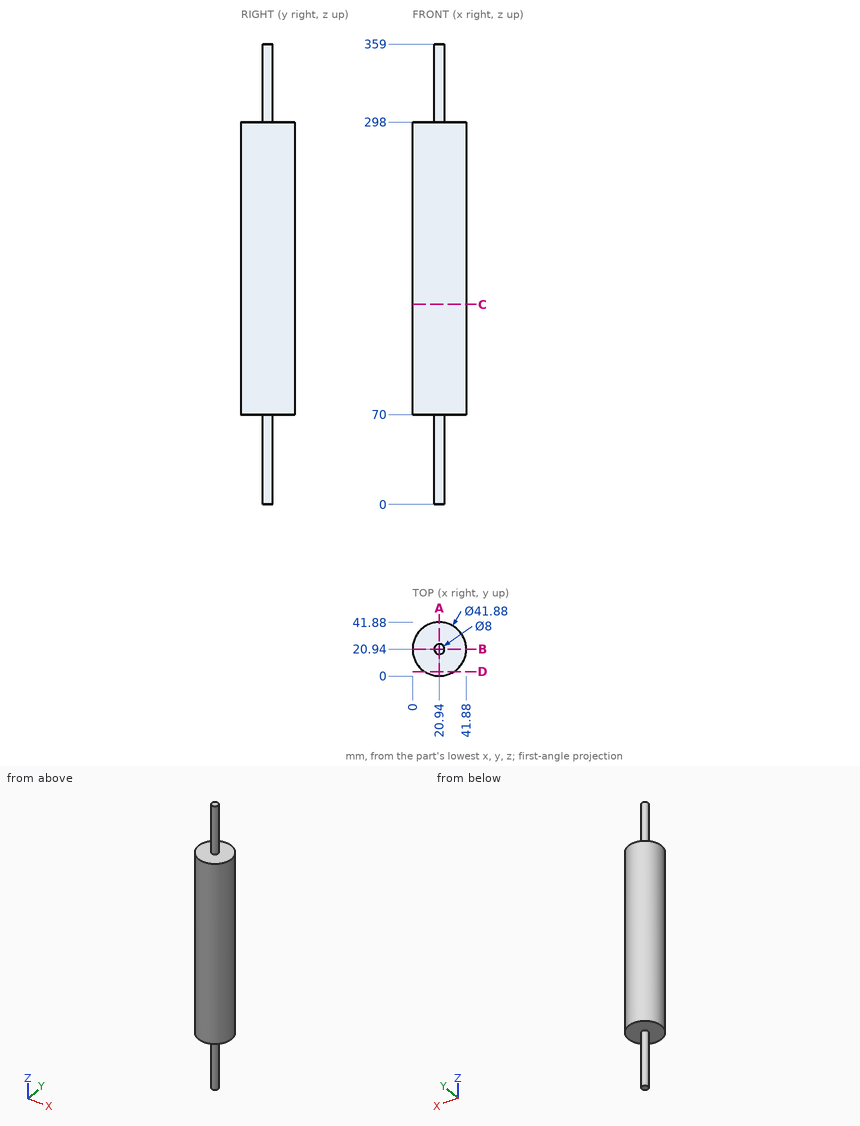
Answer from the drawing. Dimensions are ordinates in mm from the lowest x, y and z of the part. Give positions to 0.01 mm unless a question says otherwise; leave off trailing zeros. Write each loop counter-clockwise with the first axis right and the second up, starting at its lowest first coordinate (ties: lowest second). Pieces come first, ordered by that corner, then holes. Notation, with made-up numbers: M -4.5,39 L 30.5,39 A22 cw 30.5,67 Z; hole C 41,61 d10. An arc over 180 degrees is marked long. Answer as CSV lines item,"result".
Q1. Given P1, Ø2, axis at x = 13, y = 13.5, coming from the -Z side; P2, Ø5, axis at x = 34, z = 191.5, coming from the +Y side; P3, Ø3, axis at x = 36.5, y = 33, coming from the +Z side, each flat-ended and moving along its own axis, determine where each tip first touches the part or whether it passes through.
A:
P1,"stops at z = 70"
P2,"stops at y = 39.02"
P3,"stops at z = 298"
Q2. Find the intervals of material crossed by probe 1 along Z at (x, y) = (21, 15); probe 2 along Y at (x, z) = (22, 180.5); probe 3 along Y at (x, z) = (24, 23), in increasing order. Write a range as [from, to].
A:
probe 1,"z = [70, 298]"
probe 2,"y = [0.03, 41.85]"
probe 3,"y = [18.36, 23.52]"
Q3. A cutting plane is placed at C-C on z = 156. Write down the section's boundary in (x, y), plus the area to 3 significant figures.
A:
outline,"C 20.94,20.94 d41.88"
area,"1,380 mm²"
Q4. A cutting plane is placed at D-D on y = 3.5. Write down the section's boundary in (x, z).
A:
outline,"M 9.35,70 L 32.53,70 L 32.53,298 L 9.35,298 Z"
Q5. A cutting plane is placed at A-A on x = 20.94. Write down the section's boundary in (y, z), plus the area to 3 significant figures.
A:
outline,"M 0,70 L 16.94,70 L 16.94,0 L 24.94,0 L 24.94,70 L 41.88,70 L 41.88,298 L 24.94,298 L 24.94,359 L 16.94,359 L 16.94,298 L 0,298 Z"
area,"10,600 mm²"
